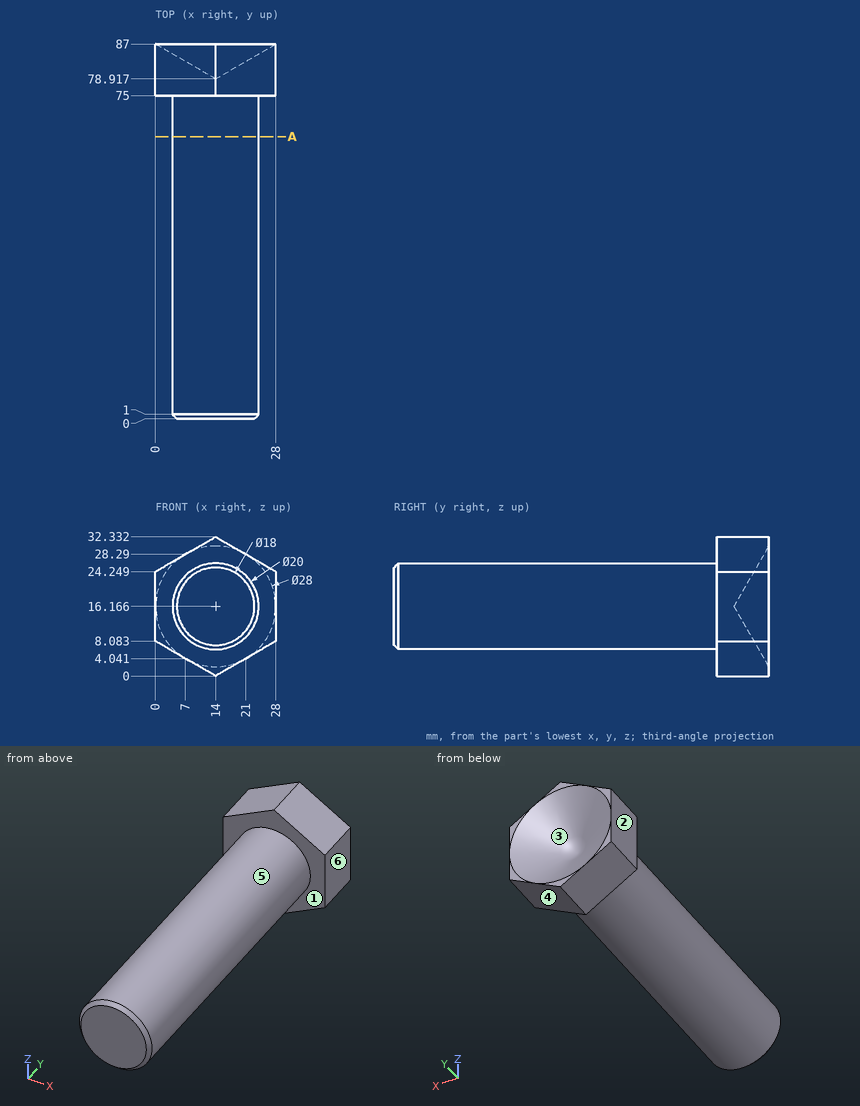
Design review of the part shown in the three views and the two pictorial views. Dimensions are in mm from the part's minimum x, y and z. A direction names the side the tool comes from. Give positions to 0.01 mm unless a question says otherwise; leave off trailing zeros. Write each loop counter-clockwise with the first axis right and the second up, starting at its lowest first coordinate (ties: lowest second). Pieces come first, ordered by that corner, then holes. Notation, with made-up numbers: M 3.5,0.5 L 18.5,0.5 A24 ccw 18.5,25.5 Z; hole C -23,-24.5 d1. An arc over 180 degrees is marked long. Return JSON: item names as keys, results as strings. Group by question number.
Item 1: Clearance check with flat-ended pins moving along their axes: pin 1 Ø3 at (x, y) = (12.5, 61) entering from -Z; pin 2 Ø5 at (x, z) = (24, 15.5) entering from +Y; pin 3 Ø5 at (y, z) = (67, 20.5) entering from -X. State where each tip first meets the part, or that it passes through.
Item 2: Tool access review of the marked faces 5 and 6: name each direction out of +Z, -Z, +X, -X, +Y, -Y from which nothing blocks a thin tool from reaching the whole face with its end or side.
Item 3: Wall thickness on line 1 along Y through (x, z) = (14.25, 30.5); line 2 along Z through (x, y) = (12, 22) (1 decimal); line 3 along Z through (x, y) = (20.75, 35) (1 decimal): over which ranges is each line inside the solid? List them lowest first.
Item 4: Take a section at A-A (y = 65.5). Give the boundary of the cut face in (x, z) (1 decimal), plus the area to 3 significant figures.
Item 5: The part is to be moulded in two halves that separate along X. For the marked faces 1, 2, 3 and 4, say which applies: pulls with the +X half, pulls with the -X half, needs draft (parallel to the pull), parting line crosses it, or undercut.
Return value:
{
 "1": {"pin 1": "stops at z = 6.17", "pin 2": "stops at y = 86.15", "pin 3": "stops at x = 4.17"},
 "2": {"face 5": "-Y", "face 6": "+Z, -Z, +X, +Y, -Y"},
 "3": {"line 1": "y = 75 to 87", "line 2": "z = 6.4 to 26", "line 3": "z = 8.8 to 23.5"},
 "4": {"outline": "C 14,16.2 d20", "area": "314 mm2"},
 "5": {"face 1": "needs draft", "face 2": "pulls with the -X half", "face 3": "undercut", "face 4": "pulls with the +X half"}
}
